Source: CAD feature listing. Evaluate the final solid. Frame: model axes, mm. Face numbers are marked on the shaded views. A direction names the side the tool comes from. Round coordinates to 2 decimals unless told otherwise and drop trailing zeros. Loops run counter-clockwise (first coordinate to the right, second up) from the corner with the lowest first, then second, coordinate; pieces in that order, holes last. Notation, with made-up numbers: (72, -28) -> (82, -28) arc R16 cw to (82, -16) -> close; hole circle Ø11 at (29.5, -19.75). An arc over 180 degrees is marked (long way). Put each result on its own line as item: value. Start each with the question number.
1. Contact query for flat-ended pins moving along their axis: pin 1 (4 mm diameter, centred on x = 1, z = -11.5, fed in from +Y); pin 2 (4.5 mm diameter, centred on y = -6.35, z = -6.35, fed in from -X) (3 decimals); pin 3 (3 mm diameter, centred on y = 6.35, z = 6.35, fed in from -X); pin 4 (4 mm diameter, centred on x = -1.5, z = -14, fed in from -Y). Output: stop coordinate, or through.
2. Set-up query: the marked faces 1, 2 and 3. Return all of +Z, -Z, +X, -X, +Y, -Y with unobstructed straight access to the full face (end or side cutting, diameter ignored); none if empty.
3. Cut plane C-C (x = 2.5). Return the cut outline in (y, z), then the cut area to 3 significant figures.
4. Draft query along Z for the marked faces 4, 5 and 6. Return one class per face: pulls with the +Z half, pulls with the -Z half, needs draft (parallel to the pull), parting line crosses it, or undercut.
5. Material intervals for L1, parallel to Z at x = -0.75, y = 15; L2, parallel to Y at x = 8, z = -6; L3, parallel to Y at x = -0.75, z = -6.35, sorted ascending.
6. Cut plane A-A (y = 0). Return the cut outline in (x, z) (3 decimals).
7. Cut plane D-D (x = -1.75). Return the cut outline in (y, z).
Autodesk Inventor part; units mm, degrees
ref_plane "YZ Plane" through (0, 0, 0) normal (1, 0, 0) x (0, 1, 0)
ref_plane "XZ Plane" through (0, 0, 0) normal (0, 1, 0) x (-1, 0, 0)
ref_plane "XY Plane" through (0, 0, 0) normal (0, 0, 1) x (1, 0, 0)
sketch "Sketch1" plane through (0, 0, 0) normal (0, 1, 0) x (-1, 0, 0)
  line L0 (0, 0) -> (3.175, 0)
  line L1 (3.175, 0) -> (3.175, -18.5)
  line L2 (3.175, -18.5) -> (0, -18.5)
  line L3 (0, -18.5) -> (0, 0)
  line L4 (0, 0) -> (-9.525, 0)
  line L5 (-9.525, 0) -> (-9.525, -14)
  line L6 (-9.525, -14) -> (0, -14)
  line L7 (0, -14) -> (0, 0)
  line L8 (5.715, 0) -> (-12.065, 0)
  point P0 (0, -14)
  dimension "d0" = 3.175
  dimension "d1" = 18.5
  dimension "d2" = 9.525
  dimension "d3" = 14
revolve "Revolution1" add sketch "Sketch1" angle 360 about axis through (-10, 0, 0) along (1, 0, 0)
sketch "Sketch2" plane through (-3.175, 0, 0) normal (-1, 0, 0) x (0, 0, 1)
  line L0 (0, 0) -> (6.35, 0)
  line L1 (6.35, 0) -> (6.35, 6.35)
  line L2 (6.35, 6.35) -> (0, 6.35)
  line L3 (0, 6.35) -> (0, 0)
  dimension "d5" = 6.35
  dimension "d6" = 6.35
hole "Hole1" at (-3.175, 6.35, 6.35) direction (1, 0, 0) diameter 5.4102 depth 6.35
hole "Hole2" at (-3.175, 6.35, 6.35) direction (1, 0, 0) diameter 3.302 depth 12.7 tip angle 118
pattern_circular "Circular Pattern1" count 2 over 360 about axis through (-10, 0, 0) along (1, 0, 0) of "Hole1", "Hole2"
fillet "Fillet1" radius 3.175 1 edges at (9.525, 0, 14)
properties part number "GL45 bottle cap insert"
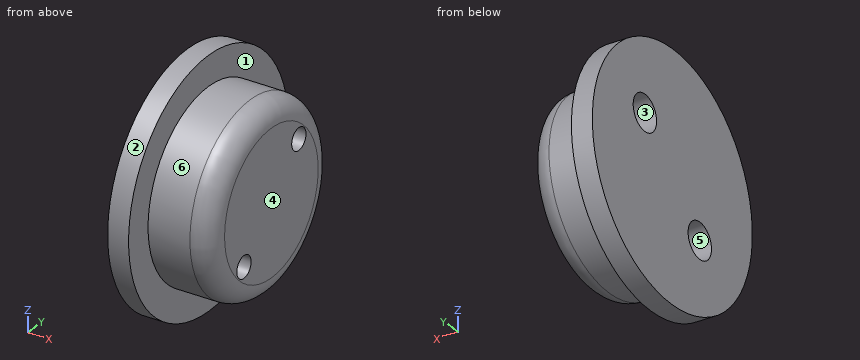
Solution:
1. pin 1: stops at y = 15.71
1. pin 2: stops at x = 3.175
1. pin 3: passes through
1. pin 4: stops at y = -14.08
2. face 1: +X
2. face 2: +X, -X
2. face 3: -X
3. outline: circle Ø28 at (0, 0); hole circle Ø5.41 at (-6.35, -6.35); hole circle Ø5.41 at (6.35, 6.35)
3. area: 570 mm^2
4. face 4: needs draft
4. face 5: undercut
4. face 6: parting line crosses it
5. L1: z = -10.83 to 10.83
5. L2: y = -12.14 to -7.96, -4.74 to 12.14
5. L3: y = -17.38 to -9.06, -3.64 to 17.38
6. outline: (-3.175, -18.5) -> (0, -18.5) -> (0, -14) -> (6.35, -14) arc R3.175 ccw to (9.525, -10.825) -> (9.525, 10.825) arc R3.175 ccw to (6.35, 14) -> (0, 14) -> (0, 18.5) -> (-3.175, 18.5) -> close
7. outline: circle Ø37 at (0, 0); hole circle Ø5.41 at (-6.35, -6.35); hole circle Ø5.41 at (6.35, 6.35)
